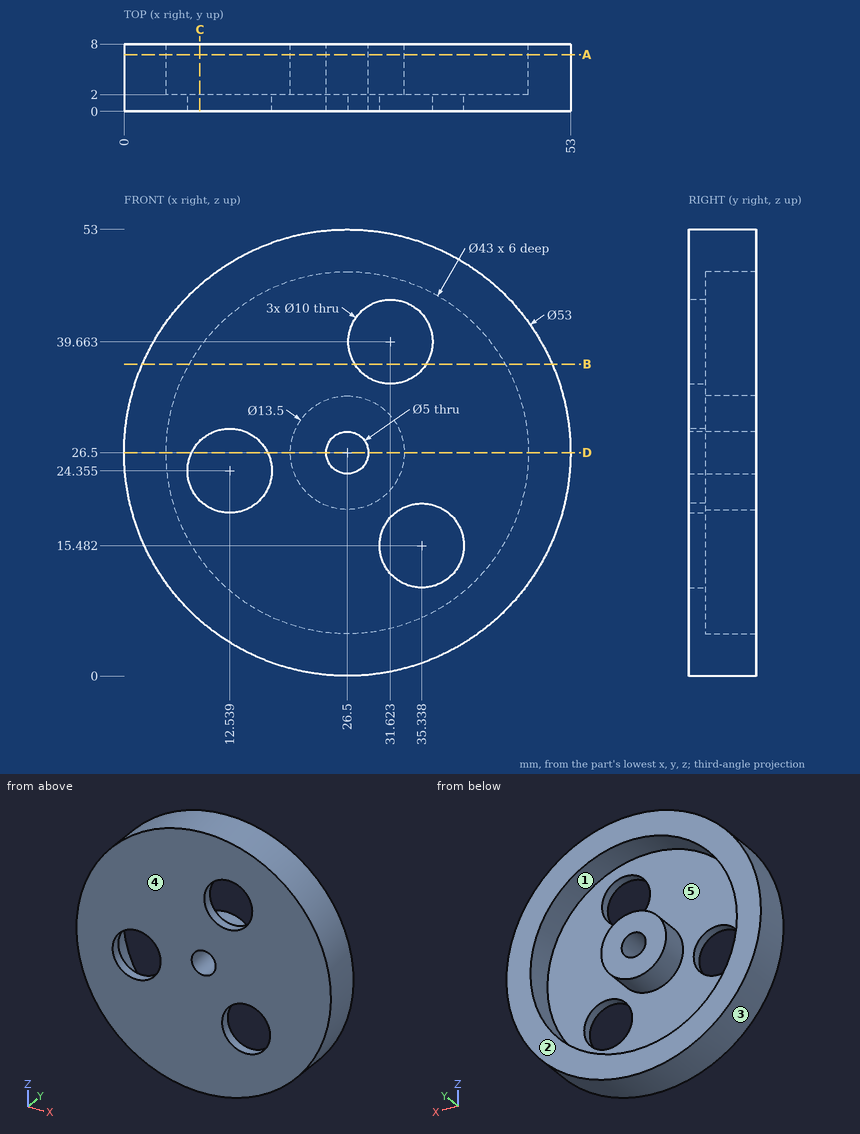
The drawing under review shows one solid part. Ordinate dimensions are in mm from its lowest x, y, z. A direction names the side the tool comes from. Give positions to 0.01 mm unless a question says otherwise; leave off trailing zeros. Write each loop counter-clockwise with the first axis right and the second up, starting at its lowest first coordinate (ties: lowest second). Pieces come first, ordered by that corner, then holes. Notation, with made-up numbers: (46.5, 45) - (85.5, 45) arc R22 ccw to (85.5, 69) - close; hole circle Ø10 at (16, -39.75). An arc over 180 degrees is marked (long way). Answer in a Markdown table with one row per item. Add a question column.
1. We need section B-B on z = 37. Write out the cut boundary in (x, y) (1 decimal), then the cut area to 3 significant figures.
2. Draft analysis for pull direction Z (two halves, no side actions). For the marked faces 1, 2 and 3, state which applies: +Z half, -Z half, draft (parallel to the pull), parting line (faces both ways), or undercut.
3. We need section C-C on x = 9. Write out the cut boundary in (y, z), then the cut area to 3 significant figures.
4. Insertion check: P1, Ø1, axis at y = 4, z = 27, coming from the +X side; P2, Ø1, axis at y = 3, z = 21, coming from the -X side; P3, Ø3, axis at y = 4.5, z = 17.5, coming from the -X side. Each pin has a flat end and moves straight along its axis. Give the tip position at first contact, or say it passes through.
5. Wall thickness on line 1 along X through (y, z) = (6.5, 26.5); line 2 along X through (y, z) = (1.5, 26.5) (1 decimal); line 3 along Z through (x, y) = (25.5, 7) (1 decimal): over which ranges is each line inside the solid? List them lowest first. Write a range as [from, to].
6. We need section D-D on z = 26.5. State how many separate pieces and enclosed holes the cut face has, then the cut area to 3 significant figures.
7. We need section A-A on y = 6.75. Write out the cut boundary in (x, z).
8. Tool access review of the marked faces 4 and 5: name each direction out of +Z, -Z, +X, -X, +Y, -Y from which nothing blocks a thin tool from reaching the whole face with its end or side.
Ans:
| question | item | result |
|---|---|---|
| 1 | outline | (2.2, 0) - (27.4, 0) - (27.4, 2) - (7.7, 2) - (7.7, 8) - (2.2, 8) - close; (35.9, 0) - (50.8, 0) - (50.8, 8) - (45.3, 8) - (45.3, 2) - (35.9, 2) - close |
| 1 | area | 147 mm^2 |
| 2 | face 1 | undercut |
| 2 | face 2 | draft |
| 2 | face 3 | parting line |
| 3 | outline | (0, 6.6) - (8, 6.6) - (8, 14.01) - (2, 14.01) - (2, 20.82) - (0, 20.82) - close; (0, 27.89) - (2, 27.89) - (2, 38.99) - (8, 38.99) - (8, 46.4) - (0, 46.4) - close |
| 3 | area | 154 mm^2 |
| 4 | P1 | stops at x = 53 |
| 4 | P2 | stops at x = 0.48 |
| 4 | P3 | stops at x = 1.08 |
| 5 | line 1 | x = [0, 5], [19.75, 24], [29, 33.25], [48, 53] |
| 5 | line 2 | x = [0, 8], [17.1, 24], [29, 53] |
| 5 | line 3 | z = [0, 5], [19.8, 24.2], [28.8, 33.2], [48, 53] |
| 6 | separate pieces | 3 |
| 6 | enclosed holes | 0 |
| 6 | area | 189 mm^2 |
| 7 | outline | circle Ø53 at (26.5, 26.5); circle Ø13.5 at (26.5, 26.5); hole circle Ø43 at (26.5, 26.5); hole circle Ø5 at (26.5, 26.5) |
| 8 | face 4 | +Z, -Z, +X, -X, -Y |
| 8 | face 5 | +Y |
